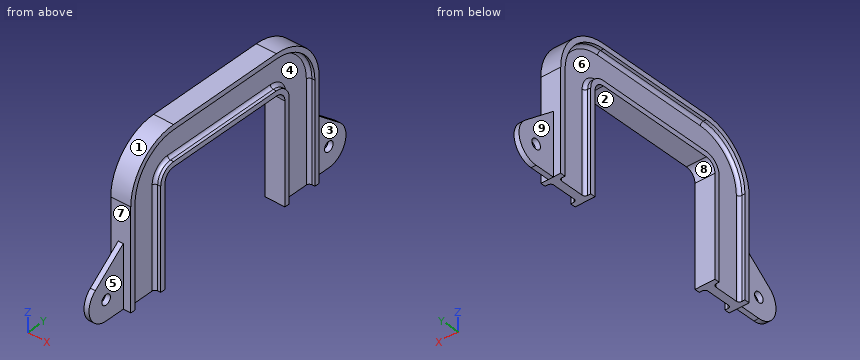
```python
from build123d import *

# Parameters (mm, degrees)
F4_R     = 5
F5_DEPTH = 2.5


with BuildPart() as f2:
    # F2: sweep along a path in F1
    with BuildLine(Plane.YZ) as f2_path:
        Line((0, 0), (60, 0))
        ThreePointArc((60, 0), (67.0710678119, -2.9289321881), (70, -10))
        Line((70, -10), (70, -110))
    # F0 (on Front) → F2 (sweep)
    with BuildSketch(Plane.XZ):
        with BuildLine():
            Line((-10, 5), (-10, 0))
            Line((-10, 0), (10, 0))
            Line((10, 0), (10, 5))
            Line((10, 5), (6.9661123479, 5))
            ThreePointArc((6.9661123479, 5), (4.8447920043, 5.8786796564), (3.9661123479, 8))
            Line((3.9661123479, 8), (3.9661123479, 32))
            ThreePointArc((3.9661123479, 32), (4.8447920043, 34.1213203436), (6.9661123479, 35))
            Line((6.9661123479, 35), (10, 35))
            Line((10, 35), (10, 40))
            Line((10, 40), (-10, 40))
            Line((-10, 40), (-10, 35))
            Line((-10, 35), (-6.9661123479, 35))
            ThreePointArc((-6.9661123479, 35), (-4.8447920043, 34.1213203436), (-3.9661123479, 32))
            Line((-3.9661123479, 32), (-3.9661123479, 8))
            ThreePointArc((-3.9661123479, 8), (-4.8447920043, 5.8786796564), (-6.9661123479, 5))
            Line((-6.9661123479, 5), (-10, 5))
        make_face()
    sweep(path=f2_path.line)

    # F3: F2 across plane


with BuildPart() as f2_1:
    add(f2.part)
    add(f2.part.mirror(Plane.XZ))

    # F4 (on Right) → F5 (join, symmetric)
    with BuildSketch(Plane.YZ):
        with BuildLine():
            Line((100, -40), (100, -110))
            Line((100, -110), (130, -110))
            ThreePointArc((130, -110), (148.8541892248, -96.6722971064), (142.5800752207, -74.4519548676))
            Line((142.5800752207, -74.4519548676), (100, -40))
        make_face()
        with Locations((130, -90)):
            Circle(F4_R, mode=Mode.SUBTRACT)
    extrude(amount=F5_DEPTH, both=True)

    # F6: F2 across plane


with BuildPart() as f2_2:
    add(f2_1.part)
    add(f2_1.part.mirror(Plane.XZ))


solid = f2_2.part
```
Can you work these out from the model? Positions are in its coordinate system, mm. Face numbers are marked on the shaded views. A direction names the side the tool comes from. Coordinates: 2 decimals unless noted, no trailing zeros. Loops run counter-clockwise (first coordinate to the right, second up) from the corner with the lowest first, then second, coordinate; pieces in that order, holes last.
Item 1: I'm going to push flat-ended pins straight in: pin 1 (12 mm diameter, centred on y = 129.5, z = -81, fed in from +X); pin 2 (1 mm diameter, centred on x = -3.5, z = -2, fed in from +Y); pin 3 (10 mm diameter, centred on x = 3.5, z = -64, fed in from -Y); pin 4 (8 mm diameter, centred on y = 130, z = -90, fed in from +X). Where does each tip first touch, or does it pass through?
Answers below:
pin 1: stops at x = 2.5
pin 2: stops at y = 109.43
pin 3: stops at y = -135.72
pin 4: passes through
Item 2: Please list where these lines run through material, in increasing order: L1, parallel to Y at x = 6.5, z = -32.5; L2, parallel to Z at x = 7.75, y = 36; L3, parallel to Y at x = 2, z = -27.
Answers below:
L1: y = -110 to -104.96, -75.04 to -70, 70 to 75.04, 104.96 to 110
L2: z = 0 to 5, 35 to 40
L3: y = -110 to -70, 70 to 110
Item 3: Suppose I cut it at A-A (y = 3.5). Please give me the cut outline in (x, z), then the cut area to 3 significant figures.
Answers below:
outline: (-10, 0) - (10, 0) - (10, 5) - (6.97, 5) arc R3 cw to (3.97, 8) - (3.97, 32) arc R3 cw to (6.97, 35) - (10, 35) - (10, 40) - (-10, 40) - (-10, 35) - (-6.97, 35) arc R3 cw to (-3.97, 32) - (-3.97, 8) arc R3 cw to (-6.97, 5) - (-10, 5) - close
area: 446 mm2
Item 4: If we mould it in two halves opening along Z, with no side actions, what happens to the marked faces 1, 2, 3 and 4? For each: released by +Z, released by -Z, zero draft, split by the parting line, or undercut.
Answers below:
face 1: released by +Z
face 2: released by -Z
face 3: zero draft
face 4: undercut
Item 5: Which directions (+Z, -Z, +X, -X, +Y, -Y) give clear straight access to the entire face, cutting with the end or side of a thin tool? Please do the marked faces 5, 6, 7, 8 and 9.
Answers below:
face 5: +Z, -Z, +X, -Y
face 6: -X
face 7: +Z, -Y
face 8: -Z, +X, -X
face 9: +Z, -Z, -X, +Y
Item 6: Suppose I cut it at B-B (z = -90). State how many separate pieces and enclosed holes the cut face has, then the cut area to 3 significant figures.
Answers below:
separate pieces: 4
enclosed holes: 0
area: 1,190 mm2
